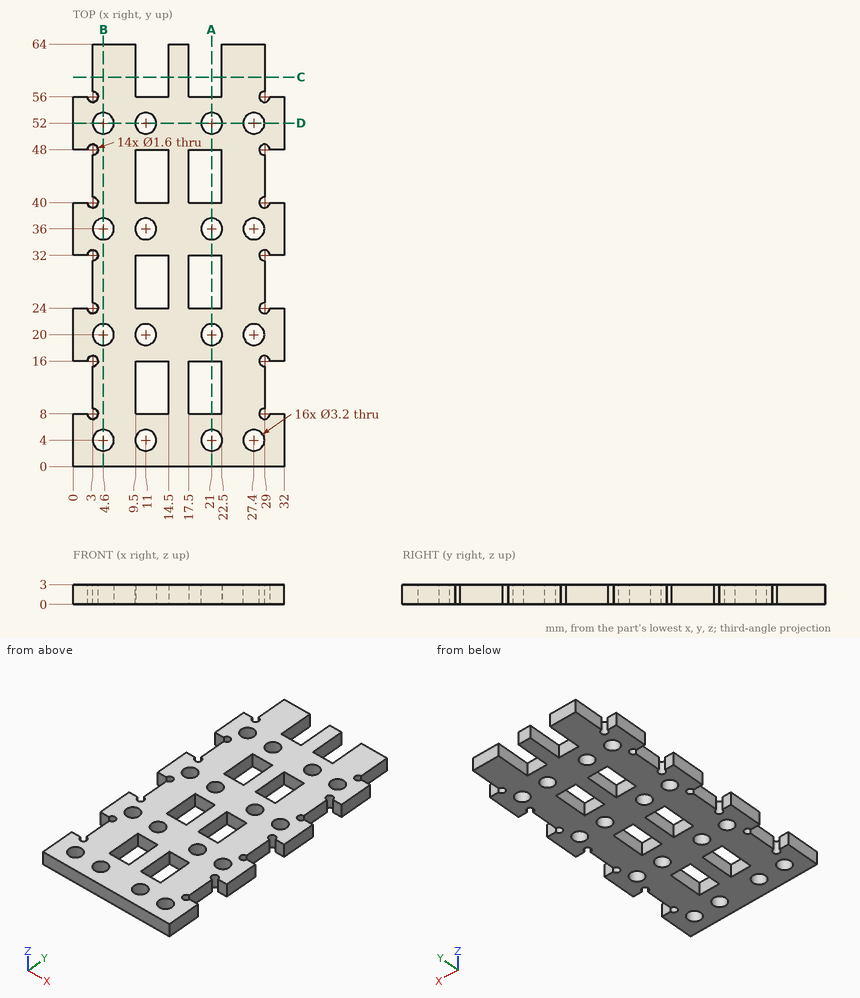
Geometry: see drawing. Coordinates: mm, zero at the bounding-box minimum. Give positions to 0.01 mm unless a question says otherwise; leave off trailing zeros. Order: outer loops, then holes, each group sorted by start corner. A loop starts at its lowest first (then second) coordinate and runs counter-clockwise, first axis right, second up. Notation, with made-up numbers: M -38,65 L -31,65 A8 cw -31,75 Z; hole C 49.25,-36 d5. An arc over 180 degrees is marked long. Answer as a JSON object with one key per item and string values.
1. Cut plane A-A, the plane x = 21. State how many separate pieces and enclosed holes the cut face has, and give its area (3 significant figures).
Result sheet:
{"separate pieces": "8", "enclosed holes": "0", "area": "57.6 mm²"}
2. Cut plane D-D, the plane y = 52. Output: boundary loops of the cut face in (x, z), and give its area (3 significant figures).
Result sheet:
{"outline": "M 0,0 L 3,0 L 3,3 L 0,3 Z; M 6.2,0 L 9.4,0 L 9.4,3 L 6.2,3 Z; M 12.6,0 L 19.4,0 L 19.4,3 L 12.6,3 Z; M 22.6,0 L 25.8,0 L 25.8,3 L 22.6,3 Z; M 29,0 L 32,0 L 32,3 L 29,3 Z", "area": "57.6 mm²"}
3. First-contact query: P1, Ø1.4, axis at x = 3, y = 40, coming from the -Z side; P2, Ø5, axis at x = 4.6, y = 20, coming from the -Z side; P3, Ø1.5, axis at y = 29.5, z = 1.5, coming from the +X side; P4, Ø0.9, axis at y = 45.5, z = 1.5, coming from the -X side. Flat tips, straight axial feed; report the tip coordinate or a pass-through.
Result sheet:
{"P1": "through", "P2": "z = 0", "P3": "x = 29", "P4": "x = 3"}
4. Cut plane B-B, the plane x = 4.6. Output: boundary loops of the cut face in (y, z).
Result sheet:
{"outline": "M 0,0 L 2.4,0 L 2.4,3 L 0,3 Z; M 5.6,0 L 18.4,0 L 18.4,3 L 5.6,3 Z; M 21.6,0 L 34.4,0 L 34.4,3 L 21.6,3 Z; M 37.6,0 L 50.4,0 L 50.4,3 L 37.6,3 Z; M 53.6,0 L 64,0 L 64,3 L 53.6,3 Z"}
5. Cut plane C-C, the plane y = 59. Output: boundary loops of the cut face in (x, z), and give its area (3 significant figures).
Result sheet:
{"outline": "M 3,0 L 9.5,0 L 9.5,3 L 3,3 Z; M 14.5,0 L 17.5,0 L 17.5,3 L 14.5,3 Z; M 22.5,0 L 29,0 L 29,3 L 22.5,3 Z", "area": "48.0 mm²"}
6. Ray query, line 1 (X direction, y = 59, z = 1.1); line 2 (Y direction, x = 18.5, z = 2.35); line 3 (Y direction, x = 4.5, z = 0.1). Return the intervals inside material, ascending. Write a range as [from, to].
Result sheet:
{"line 1": "[3, 9.5], [14.5, 17.5], [22.5, 29]", "line 2": "[0, 8], [16, 24], [32, 40], [48, 56]", "line 3": "[0, 2.4], [5.6, 18.4], [21.6, 34.4], [37.6, 50.4], [53.6, 64]"}
